from build123d import *

# Parameters (mm, degrees)
SKETCH1_W           = 93
SKETCH1_H           = 37.5
SKETCH1_R           = 1.45
BOSS_EXTRUDE1_DEPTH = 3.175


with BuildPart() as part:
    # Sketch1 → Boss-Extrude1 (new body)
    with BuildSketch(Plane(origin=(0, 0, 0), x_dir=(1, 0, 0), z_dir=(0, 1, 0))):
        with Locations((43.5, -18.75)):
            Rectangle(SKETCH1_W, SKETCH1_H)
        with Locations((85, -32.5)):
            Circle(SKETCH1_R, mode=Mode.SUBTRACT)
        with Locations((85, -22.5)):
            Circle(SKETCH1_R, mode=Mode.SUBTRACT)
        with Locations((5, -32.5)):
            Circle(SKETCH1_R, mode=Mode.SUBTRACT)
        with Locations((15, -32.5)):
            Circle(SKETCH1_R, mode=Mode.SUBTRACT)
    boss_extrude1 = extrude(amount=BOSS_EXTRUDE1_DEPTH)

    # Mirror1: Boss-Extrude1 across plane
    add(boss_extrude1.mirror(Plane(origin=(-3, 3.175, 0), x_dir=(1, 0, 0), z_dir=(0, 0, 1))))


solid = part.part
For this review, take the finished solid that the model builds, in its own axes (mm). Give positions to 0.01 mm unless a question says otherwise; leave off trailing zeros. Order: outer loops, then holes, each group sorted by start corner. A loop starts at its lowest first (then second) coordinate and runs counter-clockwise, first axis right, second up. Notation, with made-up numbers: (5, -1.75) - (60, -1.75) arc R23 cw to (60, 20.25) - close; hole circle Ø6 at (-8.5, 82.5). An arc over 180 degrees is marked (long way). Answer as a JSON object with one key per item and string values. Group by question number.
Item 1: Draft analysis for pull direction X (two halves, no side actions). For faces 1 (the flat face through (-3, 2, -1)), 2 (the cylindrical face through (3.85, 1.57, -33.38)), 3 (the cylindrical face through (85.669, 1.565, 33.786)), 4 (the flat face through (43, 2, -37.5)), state which applies: pulls with the +X half, pulls with the -X half, needs draft (parallel to the pull), parting line crosses it, or undercut.
Item 2: Take a section at A-A on x = 15. Give the boundary of the cut face in (y, z) (3 decimals).
Item 3: Take a section at B-B on z = 22.5. Give the boundary of the cut face in (x, y) (3 decimals), and give its area (3 significant figures).
Item 4: Clearance check with flat-ended pins moving along their axes: pin 1 Ø4.5 at (x, z) = (85, 32.5) entering from -Y; pin 2 Ø2.5 at (x, z) = (5, 32.5) entering from +Y. State where each tip first meets the part, or that it passes through.
Item 5: Take a section at C-C on z = 32.5. Give the boundary of the cut face in (x, y) (3 decimals).
Item 6: Wall thickness on line 1 along X through (y, z) = (2.1, 32.5); line 2 along Z through (x, y) = (15, 1.5); line 3 along Z through (x, y) = (14, 0.7): over which ranges is each line inside the solid? List them lowest first.
Reported:
{
 "1": {"face 1": "pulls with the -X half", "face 2": "undercut", "face 3": "undercut", "face 4": "needs draft"},
 "2": {"outline": "(0, -37.5) - (3.175, -37.5) - (3.175, -33.95) - (0, -33.95) - close; (0, -31.05) - (3.175, -31.05) - (3.175, 31.05) - (0, 31.05) - close; (0, 33.95) - (3.175, 33.95) - (3.175, 37.5) - (0, 37.5) - close"},
 "3": {"outline": "(-3, 0) - (83.55, 0) - (83.55, 3.175) - (-3, 3.175) - close; (86.45, 0) - (90, 0) - (90, 3.175) - (86.45, 3.175) - close", "area": "286 mm^2"},
 "4": {"pin 1": "y = 0", "pin 2": "through"},
 "5": {"outline": "(-3, 0) - (3.55, 0) - (3.55, 3.175) - (-3, 3.175) - close; (6.45, 0) - (13.55, 0) - (13.55, 3.175) - (6.45, 3.175) - close; (16.45, 0) - (83.55, 0) - (83.55, 3.175) - (16.45, 3.175) - close; (86.45, 0) - (90, 0) - (90, 3.175) - (86.45, 3.175) - close"},
 "6": {"line 1": "-3 to 3.55, 6.45 to 13.55, 16.45 to 83.55, 86.45 to 90", "line 2": "-37.5 to -33.95, -31.05 to 31.05, 33.95 to 37.5", "line 3": "-37.5 to -33.55, -31.45 to 31.45, 33.55 to 37.5"}
}
